```python
from build123d import *

# Parameters (mm, degrees)
F0_W     = 40
F0_H     = 59
F1_DEPTH = 10
F3_DEPTH = 8
F4_R     = 6
F5_DEPTH = 4
F7_DEPTH = 5
F9_DEPTH = 5


with BuildPart() as f1:
    # F0 (on Top) → F1 (new body, symmetric)
    with BuildSketch(Plane.XY):
        with Locations((0, -29.5)):
            Rectangle(F0_W, F0_H)
    extrude(amount=F1_DEPTH, both=True)

    # F2 (on face) → F3 (cut)
    with BuildSketch(Plane(origin=(0, 0, 0), x_dir=(-1, 0, 0), z_dir=(0, 1, 0))):
        with BuildLine():
            Line((-0.9, -0.8), (0.9, -0.8))
            ThreePointArc((0.9, -0.8), (1.7, 0), (0.9, 0.8))
            Line((0.9, 0.8), (-0.9, 0.8))
            ThreePointArc((-0.9, 0.8), (-1.7, 0), (-0.9, -0.8))
        make_face()
    extrude(amount=-F3_DEPTH, mode=Mode.SUBTRACT)

    # F4 (on face) → F5 (join)
    with BuildSketch(Plane.XZ.offset(59)):
        Circle(F4_R)
    extrude(amount=F5_DEPTH)

    # F6 (on face) → F7 (cut)
    with BuildSketch(Plane(origin=(-20, 0, 0), x_dir=(0, -1, 0), z_dir=(-1, 0, 0))):
        Polygon((59, -6), (0, 0.8), (0, -10), (59, -10), align=None)
    extrude(amount=-F7_DEPTH, mode=Mode.SUBTRACT)

    # F8 (on face) → F9 (cut)
    with BuildSketch(Plane.YZ.offset(20)):
        Polygon((-59, 6), (0, -0.8), (0, 10), (-59, 10), align=None)
    extrude(amount=-F9_DEPTH, mode=Mode.SUBTRACT)


solid = f1.part
```
Geometry check sheet. Reference: the model listing, model coordinates, mm. A direction names the side the tool comes from. Round coordinates to 2 decimals unless told otherwise and drop trailing zeros. Order: outer loops, then holes, each group sorted by start corner. A loop starts at its lowest first (then second) coordinate and runs counter-clockwise, first axis right, second up. Notation, with made-up numbers: (67, -27.75) - (85, -27.75) arc R31 ccw to (85, 8.25) - close; hole circle Ø5 at (77.25, 45). An arc over 180 degrees is marked (long way). Use a Markdown table: item, result. Add a question column.
(1) Sectioned sample at A-A, the plane x = 0. Enter the section's corners in (y, z).
(2) Material ranges on line 1 along Y through (x, z) = (7.5, -5); line 2 along X through (y, z) = (-14, 7.5); line 3 along X through (y, z) = (-44, -9), recorded low to high. Write a range as [from, to].
(3) Sectioned sample at B-B, the plane z = -2.25. Enter the section's corners in (x, y).
(4) Sectioned sample at C-C, the plane y = -44.5. Enter the section's corners in (x, z).
(5) Tool access check on faces 1 (the flat face through (-15, -23, -6)), 2 (the flat face through (17.535, -29.913, 2.648)), 3 (the cylindrical face through (-1.7, -3.9, 0)), 4 (the cylindrical face through (-6, -61, 0)). Record the directions out of +Z, -Z, +X, -X, +Y, -Y that give a thin tool (end or side, any length) a straight path to the whole face; none if there is none.
(6) Depth check by flat-ended pin: pin 1 (2 mm diameter, centred on y = -33, z = -7, fed in from -X); pin 2 (1 mm diameter, centred on x = 10.5, z = -2, fed in from -Y); pin 3 (5.5 mm diameter, centred on y = -17.5, z = 6.5, fed in from +X). Enter the tip coordinate at first touch or a pass-through.
(7) Release check for a two-part mould opening along Z. For faces 5 (the flat face through (-17.535, -29.913, -2.648)), 6 (the flat face through (15, -23, 6)), 7 (the flat face through (0, -4, 0.8)) record: pulls with the +Z half, pulls with the -Z half, needs draft (parallel to the pull), parting line crosses it, or undercut.
(8) Sectioned sample at D-D, the plane z = 5. Enter the section's corners in (x, y).
Answers below:
| question | item | result |
|---|---|---|
| 1 | outline | (-63, -6) - (-59, -6) - (-59, -10) - (0, -10) - (0, -0.8) - (-8, -0.8) - (-8, 0.8) - (0, 0.8) - (0, 10) - (-59, 10) - (-59, 6) - (-63, 6) - close |
| 2 | line 1 | [-59, 0] |
| 2 | line 2 | [-20, 15] |
| 2 | line 3 | [-15, 20] |
| 3 | outline | (-20, -59) - (-5.56, -59) - (-5.56, -63) - (5.56, -63) - (5.56, -59) - (20, -59) - (20, 0) - (-15, 0) - (-15, -26.46) - (-20, -26.46) - close |
| 4 | outline | (-20, -4.33) - (-15, -4.33) - (-15, -10) - (20, -10) - (20, 4.33) - (15, 4.33) - (15, 10) - (-20, 10) - close |
| 5 | face 1 | -Z, -X, +Y |
| 5 | face 2 | +Z, +X, +Y |
| 5 | face 3 | +Y |
| 5 | face 4 | -Y |
| 6 | pin 1 | x = -15 |
| 6 | pin 2 | y = -59 |
| 6 | pin 3 | x = 15 |
| 7 | face 5 | pulls with the -Z half |
| 7 | face 6 | needs draft |
| 7 | face 7 | undercut |
| 8 | outline | (-20, -59) - (-3.32, -59) - (-3.32, -63) - (3.32, -63) - (3.32, -59) - (20, -59) - (20, -50.32) - (15, -50.32) - (15, 0) - (-20, 0) - close |
